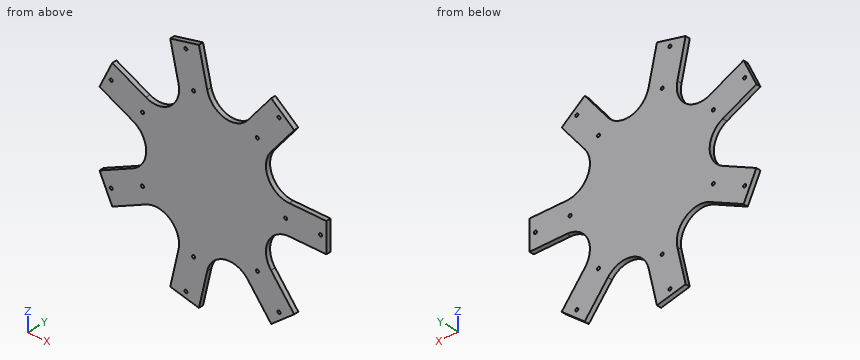
```python
from build123d import *

# Parameters (mm, degrees)
SKETCH3_W           = 250
SKETCH3_H           = 63.5
SKETCH3_R           = 3.25
BOSS_EXTRUDE1_DEPTH = 10
CIRPATTERN1_COUNT   = 7
FILLET1_R           = 50


with BuildPart() as part:
    # Sketch3 → Boss-Extrude1 (new body)
    with BuildSketch(Plane(origin=(0, 0, 0), x_dir=(1, 0, 0), z_dir=(0, 1, 0))):
        with Locations((125, 0)):
            Rectangle(SKETCH3_W, SKETCH3_H)
        with Locations((162.3, 0)):
            Circle(SKETCH3_R, mode=Mode.SUBTRACT)
        with Locations((237.3, 0)):
            Circle(SKETCH3_R, mode=Mode.SUBTRACT)
    boss_extrude1 = extrude(amount=BOSS_EXTRUDE1_DEPTH)

    # CirPattern1: Boss-Extrude1 ×7 about axis
    cirpattern1_axis = Axis((0, 0, 0), (0, 1, 0))
    for i in range(1, CIRPATTERN1_COUNT):
        add(boss_extrude1.rotate(cirpattern1_axis, i * 360 / CIRPATTERN1_COUNT))

    # Fillet1
    fillet1_edges = [part.edges().sort_by_distance(p)[0] for p in [
        (65.929554341, 5, 31.75),
        (65.929554341, 5, -31.75),
        (16.283255204, 5, 71.341602418),
        (-45.624667219, 5, 57.211523112),
        (-73.176284653, 5, 0),
        (-45.624667219, 5, -57.211523112),
        (16.283255204, 5, -71.341602418),
    ]]
    fillet(fillet1_edges, radius=FILLET1_R)


solid = part.part
```
Geometry: final body of the model. Coordinates: model frame, mm. Round coordinates to 2 decimals unless told otherwise and drop trailing zeros. Write each loop counter-clockwise with the first axis right and the second up, starting at its lowest first coordinate (ties: lowest second). Pieces come first, ordered by that corner, then holes.
Item 1: Section query C-C (x = 39.5). Return loops of the section in (y, z), plus the area to 3 significant figures.
Item 2: Material intervals for L1, parallel to Z at x = 237.3, y = 3.25; L2, parallel to Z at x = 162.3, y = 4; L3, parallel to X at y = 4.5, z = 156.5, sorted ascending.
Item 3: Pin query (flat end, axial travel): P1, Ø1, axis at x = -64.5, y = 3.5, coming from the -Z side; P2, Ø2, axis at x = -124, y = 3.5, coming from the +Z side; P3, Ø3, axis at x = 75, y = 3.5, coming from the -Z side. Return the tip coordinate at first contact, or that it passes through.
Item 4: Section query A-A (x = -199). Return loops of the section in (y, z), plus the area to 3 significant figures.
Item 5: Section query B-B (y = 3.5). Give the number of separate pieces and of enclosed holes in the cut face, plus the area to 3 significant figures.
Completed:
1. outline: (0, -133.75) - (10, -133.75) - (10, 133.75) - (0, 133.75) - close
1. area: 2,670 mm2
2. L1: z = -31.75 to -3.25, 3.25 to 31.75
2. L2: z = -190.33 to -152.59, -32.31 to -3.25, 3.25 to 32.31, 152.59 to 190.33
2. L3: x = -68.33 to -38.87, -33.36 to -0.03, 84.19 to 165.41
3. P1: stops at z = -241.82
3. P2: stops at z = 97.88
3. P3: stops at z = -147.57
4. outline: (0, -131.07) - (10, -131.07) - (10, -60.59) - (0, -60.59) - close; (0, 60.59) - (10, 60.59) - (10, 131.07) - (0, 131.07) - close
4. area: 1,410 mm2
5. separate pieces: 1
5. enclosed holes: 14
5. area: 113,000 mm2
